```python
from build123d import *

# Parameters (mm, degrees)
CYLINDER003_R             = 1.5
CYLINDER003_DEPTH         = 20
BOX037_W                  = 10
BOX037_H                  = 10
BOX037_DEPTH              = 12
FILLET013_R               = 4.5
FILLET014_R               = 4.6
FILLET014_PLACEMENT_ANGLE = 90


with BuildPart() as cylinder003:
    # Cylinder003 → Cylinder003 (new body)
    with BuildSketch(Plane(origin=(-103.2, 5, -48.3), x_dir=(1, 0, 0), z_dir=(0, 0, 1))):
        Circle(CYLINDER003_R)
    extrude(amount=CYLINDER003_DEPTH)


with BuildPart() as fillet014:
    # Box037 → Box037 (new body)
    with BuildSketch(Plane(origin=(-108.3, 0, -49.2), x_dir=(1, 0, 0), z_dir=(0, 0, 1))):
        with Locations((5, 5)):
            Rectangle(BOX037_W, BOX037_H)
    extrude(amount=BOX037_DEPTH)

    # Cut020: cut Cylinder003
    add(cylinder003.part, mode=Mode.SUBTRACT)

    # Fillet013
    fillet013_edges = [fillet014.edges().sort_by_distance(p)[0] for p in [
        (-108.3, 10, -43.2),
    ]]
    fillet(fillet013_edges, radius=FILLET013_R)

    # Fillet014
    fillet014_edges = [fillet014.edges().sort_by_distance(p)[0] for p in [
        (-108.3, 0, -43.2),
    ]]
    fillet(fillet014_edges, radius=FILLET014_R)


with BuildPart() as fillet014_1:
    # Fillet014 placement: moved
    add(fillet014.part.moved(Location((23.403045, -81.579418, 43.36))).rotate(Axis((23.403045, -81.579418, 43.36), (0, 0, -1)), FILLET014_PLACEMENT_ANGLE))


solid = fillet014_1.part
```
Input: part model. Units: mm. Frame: model coordinates. A direction names the side the tool comes from. Give positions to 0.01 mm unless a question says otherwise; leave off trailing zeros. Order: outer loops, then holes, each group sorted by start corner. A loop starts at its lowest first (then second) coordinate and runs counter-clockwise, first axis right, second up.
1. Set-up query: faces 5 (the face through (33.403, 20, 0)), 6 (the face through (28, 22, -4.94)). Return all of +Z, -Z, +X, -X, +Y, -Y with unobstructed straight access to the full face (end or side cutting, diameter ignored); none if empty.
Computed:
face 5: +Z, -Z, +X, +Y, -Y
face 6: +Z
2. Cut plane A-A (x = 27.75). Return loops of the section in (y, z).
Computed:
outline: (16.72, -5.84) - (26.71, -5.84) - (26.71, 6.16) - (22.97, 6.16) - (22.97, -4.94) - (20.27, -4.94) - (20.27, 6.16) - (16.72, 6.16) - close
3. Cut plane B-B (z = 3.5). Return loops of the section in (x, y), and give its area (3 significant figures).
Computed:
outline: (23.4, 16.72) - (33.4, 16.72) - (33.4, 22.22) arc R4.5 ccw to (28.9, 26.72) - (28, 26.72) arc R4.6 ccw to (23.4, 22.12) - close; hole circle Ø3 at (28.4, 21.62)
area: 84.0 mm2
4. Pin query (flat end, axial travel): pin 1 Ø1 at (y, z) = (25.5, -3) entering from -X. Return the tip coordinate at first contact, or that it passes through.
Computed:
pin 1: stops at x = 24.42
5. Line query: probe 1 along Y at (x, z) = (28.25, 5); probe 2 along Y at (x, z) = (29, 0.5); probe 3 along X at (y, z) = (20.5, 3.75). Output: solid intervals per line, ascending.
Computed:
probe 1: y = 16.72 to 20.13, 23.11 to 26.72
probe 2: y = 16.72 to 20.24, 23 to 26.72
probe 3: x = 23.4 to 27.41, 29.4 to 33.4
6. Draft query along X for faces 1 (the face through (28.47, 23.12, 0.53)), 2 (the face through (32.05, 25.44, 0.24)), 3 (the face through (28, 16.721, 0)), 4 (the face through (24.79, 25.41, 0.24)). Return one class per face: released by +X, released by -X, zero draft, split by the parting line, or undercut.
Computed:
face 1: undercut
face 2: released by +X
face 3: zero draft
face 4: released by -X
7. Cut plane D-D (x = 31). Return loops of the section in (y, z).
Computed:
outline: (16.72, -5.84) - (26.2, -5.84) - (26.2, 6.16) - (16.72, 6.16) - close
8. Cut plane C-C (y = 21.5). Return loops of the section in (x, z).
Computed:
outline: (23.4, -5.84) - (33.4, -5.84) - (33.4, 6.16) - (29.9, 6.16) - (29.9, -4.94) - (26.91, -4.94) - (26.91, 6.16) - (23.4, 6.16) - close
